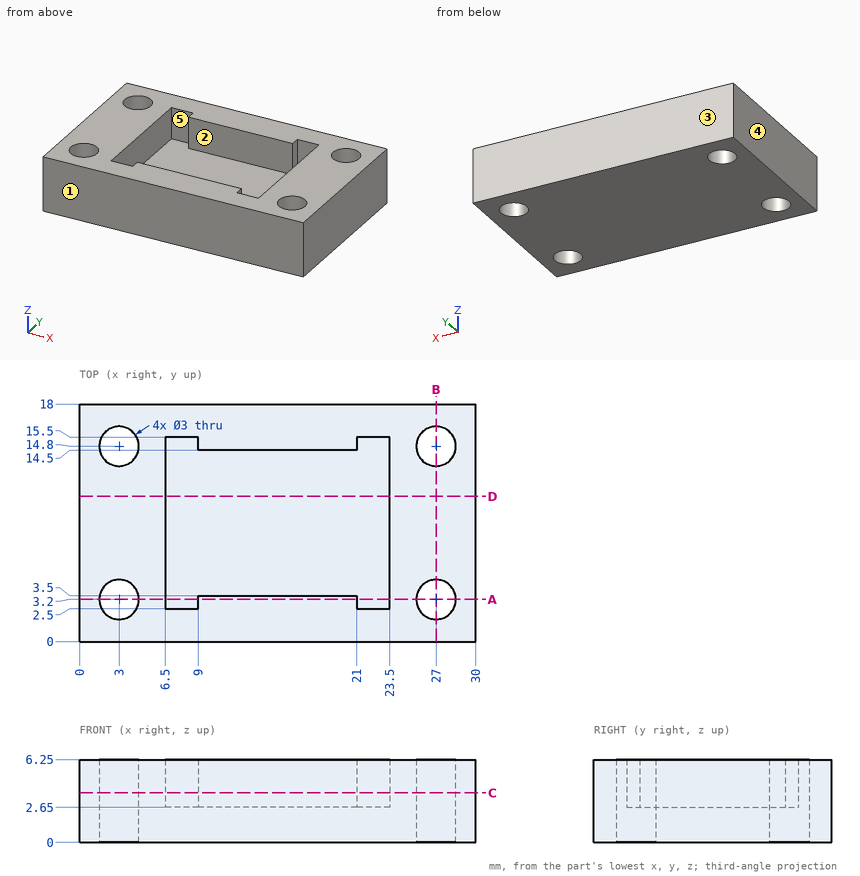
The figure shows three views and two pictorial views of one solid part (mm, origin at its lowest corner). Answer the questions. A direction names the side the tool comes from. Give positions to 0.01 mm unless a question says otherwise; leave off trailing zeros. Write each loop counter-clockwise with the first axis right and the second up, starting at its lowest first coordinate (ties: lowest second). Pieces come first, ordered by that corner, then holes. Notation, with made-up numbers: (44.5, 32.5) -> (60.5, 32.5) arc R29 cw to (60.5, 63.5) -> close; hole circle Ø10 at (24.25, -30.75). An arc over 180 degrees is marked (long way). Write each question's results on one line, items separated by ' | '.
1. Find section A-A on y = 3.2. Determine the outline of the cut face in (x, z), and give its area (3 significant figures).
Data:
outline: (0, 0) -> (1.5, 0) -> (1.5, 6.25) -> (0, 6.25) -> close; (4.5, 0) -> (25.5, 0) -> (25.5, 6.25) -> (23.5, 6.25) -> (23.5, 2.65) -> (21, 2.65) -> (21, 6.25) -> (9, 6.25) -> (9, 2.65) -> (6.5, 2.65) -> (6.5, 6.25) -> (4.5, 6.25) -> close; (28.5, 0) -> (30, 0) -> (30, 6.25) -> (28.5, 6.25) -> close | area: 132 mm^2
2. Find section C-C on z = 3.75. Determine the outline of the cut face in (x, y).
Data:
outline: (0, 0) -> (30, 0) -> (30, 18) -> (0, 18) -> close; hole circle Ø3 at (3, 3.2); hole circle Ø3 at (3, 14.8); hole (6.5, 2.5) -> (9, 2.5) -> (9, 3.5) -> (21, 3.5) -> (21, 2.5) -> (23.5, 2.5) -> (23.5, 15.5) -> (21, 15.5) -> (21, 14.5) -> (9, 14.5) -> (9, 15.5) -> (6.5, 15.5) -> close; hole circle Ø3 at (27, 3.2); hole circle Ø3 at (27, 14.8)
3. Straight lines are drawn through the part: L1, parallel to X at y = 3.25, z = 2.75; L2, parallel to Y at x = 3, z = 2; L3, parallel to X at y = 12.25, z = 5.75. For each, find the intervals that lie inside material, in ascending order.
Data:
L1: 0 to 1.5, 4.5 to 6.5, 9 to 21, 23.5 to 25.5, 28.5 to 30 | L2: 0 to 1.7, 4.7 to 13.3, 16.3 to 18 | L3: 0 to 6.5, 23.5 to 30
4. Find section B-B on x = 27. Determine the outline of the cut face in (y, z).
Data:
outline: (0, 0) -> (1.7, 0) -> (1.7, 6.25) -> (0, 6.25) -> close; (4.7, 0) -> (13.3, 0) -> (13.3, 6.25) -> (4.7, 6.25) -> close; (16.3, 0) -> (18, 0) -> (18, 6.25) -> (16.3, 6.25) -> close
5. A tool of negligible diameter and unlimited length cuts with its end or side. For the marked faces 1 and 2, from which of +Z, -Z, +X, -X, +Y, -Y can it reach the whole face along a straight path? Write none if from no direction.
Data:
face 1: +Z, -Z, +X, -X, -Y | face 2: +Z
6. Determine the mould class of the marked faces 3, 4 and 5 for opening direction X: +X half, -X half, draft (parallel to the pull), parting line (faces both ways), or undercut.
Data:
face 3: draft | face 4: -X half | face 5: undercut
7. Find section D-D on y = 11. Determine the outline of the cut face in (x, z), and give its area (3 significant figures).
Data:
outline: (0, 0) -> (30, 0) -> (30, 6.25) -> (23.5, 6.25) -> (23.5, 2.65) -> (6.5, 2.65) -> (6.5, 6.25) -> (0, 6.25) -> close | area: 126 mm^2
